Geometry: final body of the model. Coordinates: model frame, mm. A direction names the side the tool comes from. Give positions to 0.01 mm unless a question says otherwise; leave off trailing zeros. Write each loop counter-clockwise with the first axis right and the second up, starting at its lowest first coordinate (ties: lowest second). Pieces come first, ordered by that corner, then holes. Notation, with made-up numbers: (3, 9.5) -> (20, 9.5) arc R28 ccw to (20, 47.5) -> close; hole circle Ø1 at (-31, 26.25). An arc over 180 degrees is marked (long way). Use CSV: the item, a comma, the result in double quotes. Start each with the question number.
1) Contact query for flat-ended pins moving along their axis: P1, Ø1.5, axis at x = -26, y = 26, coming from the -Z side; P2, Ø10.5, axis at x = -27.5, z = -64.5, coming from the +Y side; P3, Ø10, axis at x = -20, z = -22.5, coming from the +Y side. Output: stop coordinate, or through.
2) Section B-B (x = 10). Output: boundary loops of the cut face in (y, z), plus the area to 3 significant figures.
3) Material intervals for line 1 (Z direction, x = -10, y = 32); line 2 (Z direction, x = -4.5, y = -13.5); line 3 (Y direction, x = 4.5, z = -56.5), sorted ascending. Write a range as [from, to].
4) Section C-C (y = 30). Output: boundary loops of the cut face in (x, z).
5) Set-up query: faces 1 (the face through (10, -12, -20)), 2 (the face through (-8, 18.99, -16)), 3 (the face through (-29, 8.99, -62)), 4 (the face through (-25, 26, -10)). Return all of +Z, -Z, +X, -X, +Y, -Y with unobstructed straight access to the full face (end or side cutting, diameter ignored); none if empty.
6) Section A-A (z = -31.5). Output: boundary loops of the cut face in (x, y).
7) Section D-D (z = -68). Output: boundary loops of the cut face in (x, y).
8) Draft query along Z for faces 5 (the face through (-8, 33.99, -112)), 6 (the face through (-22, 24, -45)), 7 (the face through (-15, 27, -5)). Return one class per face: pulls with the +Z half, pulls with the -Z half, needs draft (parallel to the pull), parting line crosses it, or undercut.
```python
from build123d import *

# Parameters (mm, degrees)
BOSS_EXTRUDE1_DEPTH      = 115
CUT_EXTRUDE4_DEPTH       = 115
CUT_EXTRUDE5_DEPTH       = 115
CUT_EXTRUDE7_DEPTH       = 15
SKETCH8_W                = 35
SKETCH8_H                = 40
CUT_EXTRUDE8_DEPTH       = 55
BOSS_EXTRUDE2_DEPTH      = 10
BOSS_EXTRUDE2_DEPTH_BACK = 30
SKETCH9_W                = 20
SKETCH9_H                = 15
BOSS_EXTRUDE4_DEPTH      = 10
BOSS_EXTRUDE4_DEPTH_BACK = 35
SKETCH10_W               = 15
SKETCH10_H               = 15
SKETCH10_W_2             = 5
CUT_EXTRUDE9_DEPTH       = 35


with BuildPart() as part:
    # Sketch1 → Boss-Extrude1 (new body)
    with BuildSketch(Plane.XY):
        with BuildLine():
            Line((0, 50), (0, -5))
            Line((0, -5), (20, -5))
            Line((20, -5), (20, -20))
            Line((20, -20), (0, -20))
            Line((0, -20), (0, -50))
            ThreePointArc((0, -50), (-50, 0), (0, 50))
        make_face()
    extrude(amount=-BOSS_EXTRUDE1_DEPTH)

    # Sketch2 → Cut-Extrude4 (cut)
    with BuildSketch(Plane.XY):
        with BuildLine():
            Line((0, -5), (-5, -5))
            ThreePointArc((-5, -5), (-8.535533906, -3.535533906), (-10, 0))
            Line((-10, 0), (-10, 48.989794856))
            ThreePointArc((-10, 48.989794856), (-5.0254481, 49.74680765), (0, 50))
            Line((0, 50), (0, -5))
        make_face()
    extrude(amount=-CUT_EXTRUDE4_DEPTH, mode=Mode.SUBTRACT)

    # Sketch6 → Cut-Extrude5 (cut)
    with BuildSketch(Plane.XY):
        with BuildLine():
            Line((0, -20), (-20, -20))
            Line((-20, -20), (-20, -45.82575695))
            ThreePointArc((-20, -45.82575695), (-10.215482184, -48.945315647), (0, -50))
            Line((0, -50), (0, -20))
        make_face()
    extrude(amount=-CUT_EXTRUDE5_DEPTH, mode=Mode.SUBTRACT)

    # Sketch7 → Cut-Extrude7 (cut)
    with BuildSketch(Plane.XY):
        with BuildLine():
            Line((20, -5), (-5, -5))
            ThreePointArc((-5, -5), (-8.535533906, -3.535533906), (-10, 0))
            Line((-10, 0), (-10, 48.989794856))
            ThreePointArc((-10, 48.989794856), (-43.080253734, 25.378962513), (-47.696960071, -15))
            Line((-47.696960071, -15), (20, -15))
            Line((20, -15), (20, -5))
        make_face()
    extrude(amount=-CUT_EXTRUDE7_DEPTH, mode=Mode.SUBTRACT)

    # Sketch8 → Cut-Extrude8 (cut)
    with BuildSketch(Plane(origin=(-10, 0, 0), x_dir=(0, 0, -1), z_dir=(1, 0, 0))):
        with Locations((62.5, 28.989794856)):
            Rectangle(SKETCH8_W, SKETCH8_H)
    extrude(amount=-CUT_EXTRUDE8_DEPTH, mode=Mode.SUBTRACT)

    # Sketch9 → Boss-Extrude2 (add, two sides: drawn at the far end of the back side and taken through both)
    with BuildSketch(Plane.XY.offset(-15).offset(-BOSS_EXTRUDE2_DEPTH_BACK)):
        with Locations((-15, 26.489794856)):
            Rectangle(SKETCH9_W, SKETCH9_H)
    extrude(amount=BOSS_EXTRUDE2_DEPTH + BOSS_EXTRUDE2_DEPTH_BACK)

    # Sketch10 → Boss-Extrude4 (add, two sides: drawn at the far end of the back side and taken through both)
    with BuildSketch(Plane(origin=(0, 0, -115), x_dir=(-1, 0, 0), z_dir=(0, 0, -1)).offset(-BOSS_EXTRUDE4_DEPTH_BACK)):
        with Locations((17.5, 26.489794856)):
            Rectangle(SKETCH10_W, SKETCH10_H)
        with Locations((7.5, 26.489794856)):
            Rectangle(SKETCH10_W_2, SKETCH10_H)
    extrude(amount=BOSS_EXTRUDE4_DEPTH + BOSS_EXTRUDE4_DEPTH_BACK)

    # Sketch11 → Cut-Extrude9 (cut)
    with BuildSketch(Plane(origin=(0, -5, 0), x_dir=(1, 0, 0), z_dir=(0, 1, 0))):
        with BuildLine():
            Line((5, 105), (5, 25))
            ThreePointArc((5, 25), (10, 20), (15, 25))
            Line((15, 25), (15, 105))
            ThreePointArc((15, 105), (10, 110), (5, 105))
        make_face()
    extrude(amount=-CUT_EXTRUDE9_DEPTH, mode=Mode.SUBTRACT)


solid = part.part
```
Answers follow:
1,P1,"stops at z = -115"
1,P2,"stops at y = 8.99"
1,P3,"stops at y = 47.7"
2,outline,"(-20, -115) -> (-5, -115) -> (-5, -110) -> (-20, -110) -> close; (-20, -20) -> (-5, -20) -> (-5, -15) -> (-15, -15) -> (-15, 0) -> (-20, 0) -> close"
2,area,"225 mm^2"
3,line 1,"z = [-125, -80], [-45, -5]"
3,line 2,"z = [-115, -15]"
3,line 3,"y = [-20, -5]"
4,outline,"(-40, -115) -> (-25, -115) -> (-25, -125) -> (-5, -125) -> (-5, -80) -> (-40, -80) -> close; (-40, -45) -> (-5, -45) -> (-5, -5) -> (-25, -5) -> (-25, -15) -> (-40, -15) -> close"
5,face 1,"+Y, -Y"
5,face 2,"+Z, +X"
5,face 3,"+X, -X, +Y"
5,face 4,"+Z, -X, +Y"
6,outline,"(-20, -45.83) -> (-20, -20) -> (5, -20) -> (5, -5) -> (-5, -5) arc R5 cw to (-10, 0) -> (-10, 18.99) -> (-5, 18.99) -> (-5, 33.99) -> (-10, 33.99) -> (-10, 48.99) arc R50 ccw to start; (15, -20) -> (20, -20) -> (20, -5) -> (15, -5) -> close"
7,outline,"(-49.19, 8.99) arc R50 ccw to (-20, -45.83) -> (-20, -20) -> (5, -20) -> (5, -5) -> (-5, -5) arc R5 cw to (-10, 0) -> (-10, 8.99) -> close; (15, -20) -> (20, -20) -> (20, -5) -> (15, -5) -> close"
8,face 5,"needs draft"
8,face 6,"undercut"
8,face 7,"pulls with the +Z half"
